from build123d import *

# Parameters (mm, degrees)
F0_W      = 30
F0_H      = 15
F1_DEPTH  = 4.5
F3_DEPTH  = 30
F4_W      = 9.5
F4_H      = 2
F4_W_2    = 2
F4_W_3    = 11
F5_DEPTH  = 25
F6_R      = 1.025
F7_DEPTH  = 30
F8_W      = 9.5
F8_H      = 2
F9_DEPTH  = 25
F10_W     = 11
F10_H     = 2
F11_DEPTH = 25
F12_W     = 2
F12_H     = 2
F13_DEPTH = 25
F15_DEPTH = 0.5
F16_W     = 5
F16_H     = 13
F16_H_2   = 3.8236103207
F17_DEPTH = 0.5
F18_W     = 2
F18_H     = 14.3228756555
F19_DEPTH = 3
F20_SIZE  = 2.99999
F21_SIZE  = 3
F22_SIZE  = 0.5
F23_SIZE  = 0.49999
F25_DEPTH = 3


# Not quite as in the source:
# - a fillet or chamfer is up to 0.001 mm smaller than in the source, because OpenCascade refuses the exact size
# - a feature names something its author has since deleted; it is built from what else it names


with BuildPart() as f1:
    # F0 (on Top) → F1 (new body)
    with BuildSketch(Plane.XY):
        Rectangle(F0_W, F0_H)
    extrude(amount=F1_DEPTH)

    # F2 (on face) → F3 (join)
    with BuildSketch(Plane(origin=(-15, 0, 0), x_dir=(0, -1, 0), z_dir=(-1, 0, 0))):
        with BuildLine():
            ThreePointArc((-7.5, 0.5), (-6.0857864376, 1.0857864376), (-5.5, 2.5))
            ThreePointArc((-5.5, 2.5), (-6.0857864376, 3.9142135624), (-7.5, 4.5))
            Line((-7.5, 4.5), (-7.5, 0.5))
        make_face()
        with BuildLine():
            Line((-7.5, 0.5), (-7.5, 4.5))
            ThreePointArc((-7.5, 4.5), (-9.5, 2.5), (-7.5, 0.5))
        make_face()
        with BuildLine():
            ThreePointArc((9.5, 2.5), (8.9142135624, 3.9142135624), (7.5, 4.5))
            Line((7.5, 4.5), (7.5, 0.5))
            ThreePointArc((7.5, 0.5), (8.9142135624, 1.0857864376), (9.5, 2.5))
        make_face()
    extrude(amount=-F3_DEPTH)

    # F4 (on face) → F5 (cut)
    with BuildSketch(Plane.XY.offset(4.5)):
        with Locations((-10.25, -8.5)):
            Rectangle(F4_W, F4_H)
        with Locations((10.25, -8.5)):
            Rectangle(F4_W, F4_H)
        with Locations((-14, 8.5)):
            Rectangle(F4_W_2, F4_H)
        with Locations((14, 8.5)):
            Rectangle(F4_W_2, F4_H)
        with Locations((0, 8.5)):
            Rectangle(F4_W_3, F4_H)
    extrude(amount=-F5_DEPTH, mode=Mode.SUBTRACT)

    # F6 (on face) → F7 (cut)
    with BuildSketch(Plane.YZ.offset(15)):
        with Locations((-7.5, 2.5)):
            Circle(F6_R)
        with Locations((7.5, 2.5)):
            Circle(F6_R)
    extrude(amount=-F7_DEPTH, mode=Mode.SUBTRACT)

    # F8 (on face) → F9 (cut)
    with BuildSketch(Plane.XY.offset(4.5)):
        with Locations((-10.25, -6.5)):
            Rectangle(F8_W, F8_H)
        with Locations((10.25, -6.5)):
            Rectangle(F8_W, F8_H)
    extrude(amount=-F9_DEPTH, mode=Mode.SUBTRACT)

    # F10 (on face) → F11 (cut)
    with BuildSketch(Plane.XY.offset(4.5)):
        with Locations((0, 6.5)):
            Rectangle(F10_W, F10_H)
    extrude(amount=-F11_DEPTH, mode=Mode.SUBTRACT)

    # F12 (on face) → F13 (cut)
    with BuildSketch(Plane.XY.offset(4.5)):
        with Locations((-14, 6.5)):
            Rectangle(F12_W, F12_H)
        with Locations((14, 6.5)):
            Rectangle(F12_W, F12_H)
    extrude(amount=-F13_DEPTH, mode=Mode.SUBTRACT)

    # F14 (on face) → F15 (cut)
    with BuildSketch(Plane(origin=(0, 0, 0), x_dir=(1, 0, 0), z_dir=(0, 0, -1))):
        Polygon((3, 5.5), (0, 5.5), (-3, 5.5), (-15, 0), (-15, -5.5), (-3, 0), (3, 0), (15, -5.5), (15, 0), align=None)
        Polygon((-15, 5.5), (-15, 2.75), (-9, 5.5), align=None)
        Polygon((9, 5.5), (15, 2.75), (15, 5.5), align=None)
        Polygon((-3, -2.75), (-13, -7.3333333333), (-13, -7.5), (-5.5, -7.5), (-5.5, -5.5), (5.5, -5.5), (5.5, -7.5), (13, -7.5), (13, -7.3333333333), (3, -2.75), align=None)
        Polygon((-5.5, 7.5), (-5.5, 7.1041666667), (-4.6363636364, 7.5), align=None)
        Polygon((4.6363636364, 7.5), (5.5, 7.1041666667), (5.5, 7.5), align=None)
    extrude(amount=-F15_DEPTH, mode=Mode.SUBTRACT)

    # F16 (on face) → F17 (cut)
    with BuildSketch(Plane.XY.offset(4.5)):
        with Locations((0, -1)):
            Rectangle(F16_W, F16_H)
        with Locations((0, -9.4118051603)):
            Rectangle(F16_W, F16_H_2)
    extrude(amount=-F17_DEPTH, mode=Mode.SUBTRACT)

    # F18 (on face) → F19 (join)
    with BuildSketch(Plane.XY.offset(4)):
        with Locations((0, -1.6614378278)):
            Rectangle(F18_W, F18_H)
    extrude(amount=F19_DEPTH)

    # F20 (size 3 in the source; OpenCascade refuses exactly that, so slightly less here)
    f20_edges = [f1.edges().sort_by_distance(p)[0] for p in [
        (0, -8.822876, 7),
    ]]
    chamfer(f20_edges, length=F20_SIZE)

    # F21
    f21_edges = [f1.edges().sort_by_distance(p)[0] for p in [
        (0, 5.5, 7),
    ]]
    chamfer(f21_edges, length=F21_SIZE)

    # F22
    f22_edges = [f1.edges().sort_by_distance(p)[0] for p in [
        (-1, -1.661443, 7),
        (1, -1.661443, 7),
    ]]
    chamfer(f22_edges, length=F22_SIZE)

    # F23 (size 0.5 in the source; OpenCascade refuses exactly that, so slightly less here)
    f23_edges = [f1.edges().sort_by_distance(p)[0] for p in [
        (2.5, -1, 4.5),
        (-2.5, -1, 4.5),
    ]]
    chamfer(f23_edges, length=F23_SIZE)

    # F24 (on face) → F25 (cut)
    with BuildSketch(Plane.YZ.offset(1)):
        Polygon((-5, 7), (-4.5, 6.5), (1.5, 6.5), (2, 7), align=None)
        Polygon((-4.5, 6.5), (-2, 4), (-1.5, 4), (-1, 4), (1.5, 6.5), align=None)
    extrude(amount=-F25_DEPTH, mode=Mode.SUBTRACT)


solid = f1.part
The model under review builds one solid part; all positions refer to its coordinate system, in mm. A direction names the side the tool comes from. Round coordinates to 2 decimals unless told otherwise and drop trailing zeros. Write each loop counter-clockwise with the first axis right and the second up, starting at its lowest first coordinate (ties: lowest second). Pieces come first, ordered by that corner, then holes. Notation, with made-up numbers: M 87.5,-38.5 L 105.5,-38.5 A14 ccw 105.5,-14.5 Z; hole C -8.5,49 d7. An arc over 180 degrees is marked long. Use a Markdown table: item, result. Add a question column.
Q1. To check wall thickness, follow line 1 (Z direction, x = 11.25, y = 7.5) (3 decimals); line 2 (Y direction, x = 9, z = 2.5) (3 decimals); line 3 (X direction, y = 0.75, z = 5.25). State the ranges of each line that lie inside material, in increasing order.
Q2. Machinability: for faces 4 (the face through (10, -5.5, 2)), 5 (the face through (14, 5.5, 2)), 6 (the face through (-12.042, -4.106, 0.246)), which of the approach directions +Z, -Z, +X, -X, +Y, -Y give a long, thin tool a straight path to every point of the face, cutting with its end or side? Answer none if there is none.
Q3. We need section B-B, the plane y = 7. State the section outline as (x, z) points.
Q4. We need section C-C, the plane x = -11.25. State the section outline as (y, z) points (3 decimals).
Q5. Insertion check: pin 1 (1 mm diameter, centred on x = -7, y = 3, fed in from +Z); pin 2 (0.8 mm diameter, centred on y = -4, z = 5, fed in from +X); pin 3 (1.5 mm diameter, centred on x = -4, y = 6.5, fed in from +Z); pin 4 (2.5 mm diameter, centred on y = 7.5, z = 2.5, fed in from -X). Each pin has a flat end and moves straight along its axis. Give the tip position at first contact, or say it passes through.
Q6. The part is to be moulded in two halves that separate along Y. For faces 1 (the face through (9.302, 6.476, 2.545)), 2 (the face through (-9, 0, 4.5)), 3 (the face through (-7.93, 5.01, 0.25)), say which applies: pulls with the +Y half, pulls with the -Y half, needs draft (parallel to the pull), parting line crosses it, or undercut.
Q7. We need section A-A, the plane z = 5.25. State the section outline as (x, y) points.
Findings below:
| question | item | result |
|---|---|---|
| 1 | line 1 | z = 0.5 to 1.475, 3.525 to 4.5 |
| 1 | line 2 | y = -5.5 to 6.475, 8.525 to 9.5 |
| 1 | line 3 | x = -1 to 1 |
| 2 | face 4 | +Z, -Z, +X, -Y |
| 2 | face 5 | +Z, -Z, +X, +Y |
| 2 | face 6 | -Z, -X, -Y |
| 3 | outline | M -13,0 L -12.27,0 L -12.27,0.5 L -5.5,0.5 L -5.5,1.61 L -13,1.61 Z; M -13,3.39 L -5.5,3.39 L -5.5,4.5 L -13,4.5 Z; M 5.5,0.5 L 12.27,0.5 L 12.27,0 L 13,0 L 13,1.61 L 5.5,1.61 Z; M 5.5,3.39 L 13,3.39 L 13,4.5 L 5.5,4.5 Z |
| 4 | outline | M -5.5,0.5 L -4.469,0.5 L -4.469,0 L -1.719,0 L -1.719,0.5 L 3.781,0.5 L 3.781,0 L 6.531,0 L 6.531,0.5 L 7.5,0.5 A2 ccw 7.5,4.5 L -5.5,4.5 Z; hole C 7.5,2.5 d2.05 |
| 5 | pin 1 | stops at z = 4.5 |
| 5 | pin 2 | stops at x = 1 |
| 5 | pin 3 | passes through |
| 5 | pin 4 | stops at x = -13 |
| 6 | face 1 | undercut |
| 6 | face 2 | needs draft |
| 6 | face 3 | pulls with the +Y half |
| 7 | outline | M -1,-7.57 L 1,-7.57 L 1,-3.25 L -1,-3.25 Z; M -1,0.25 L 1,0.25 L 1,4.25 L -1,4.25 Z |
